Geometry check sheet. Reference: the model listing, model coordinates, mm. Round coordinates to 2 decimals unless told otherwise and drop trailing zeros. Write each loop counter-clockwise with the first axis right and the second up, starting at its lowest first coordinate (ties: lowest second). Pieces come first, ordered by that corner, then holes. Notation, with made-up numbers: (15.25, 15) -> (50.25, 15) arc R16 cw to (50.25, 45) -> close; hole circle Ø8 at (71, 17.5). An arc over 180 degrees is marked (long way). Use a Markdown table: item, result.
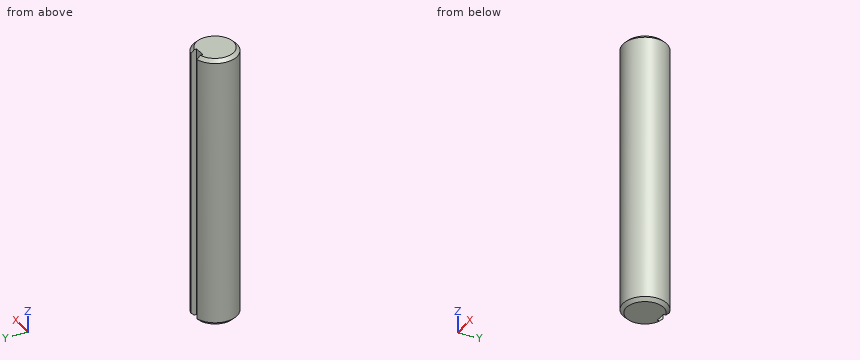
```python
from build123d import *

# Parameters (mm, degrees)
SKETCH1_R           = 4
EXTRUDE1_DEPTH      = 25
CHAMFER1_SIZE       = 0.6
SKETCH3_W           = 2
SKETCH3_H           = 1.2
EXTRUDE2_DEPTH      = 26
EXTRUDE2_DEPTH_BACK = 26


with BuildPart() as part:
    # Sketch1 → Extrude1 (new body, symmetric)
    with BuildSketch(Plane.XY):
        Circle(SKETCH1_R)
    extrude(amount=EXTRUDE1_DEPTH, both=True)

    # Chamfer1
    chamfer1_edges = [part.edges().sort_by_distance(p)[0] for p in [
        (-4, 0, -25),
        (-4, 0, 25),
    ]]
    chamfer(chamfer1_edges, length=CHAMFER1_SIZE)

    # Sketch3 → Extrude2 (cut, two sides)
    with BuildSketch(Plane.XY) as extrude2_sk:
        with Locations((0, 3.4)):
            Rectangle(SKETCH3_W, SKETCH3_H)
    extrude(amount=EXTRUDE2_DEPTH, mode=Mode.SUBTRACT)
    extrude(extrude2_sk.sketch, amount=-EXTRUDE2_DEPTH_BACK, mode=Mode.SUBTRACT)


solid = part.part
```
(1) Section check B-B on z = -8. Record the cut outline in (x, y).
A:
| item | result |
|---|---|
| outline | (-1, 2.8) -> (-1, 3.87) arc R4 ccw (long way) to (1, 3.87) -> (1, 2.8) -> close |
(2) Thickness scan on line 1 (Y direction, x = 0.25, z = 20); line 2 (X direction, y = -1, z = -6); line 3 (X direction, y = 3, z = -21.5). Record the ranges inside material, lowest first.
A:
| item | result |
|---|---|
| line 1 | y = -3.99 to 2.8 |
| line 2 | x = -3.87 to 3.87 |
| line 3 | x = -2.65 to -1, 1 to 2.65 |
(3) Gauge pin test, flat ends, axial feed: pin 1 Ø1.5 at (y, z) = (-2.5, 17) entering from -X; pin 2 Ø3 at (y, z) = (-3, -14.5) entering from +X; pin 3 Ø1.2 at (y, z) = (3.5, -2) entering from -X (3 decimals). Record the tip position at first contact, or that the pin passes through.
A:
| item | result |
|---|---|
| pin 1 | stops at x = -3.6 |
| pin 2 | stops at x = 3.71 |
| pin 3 | stops at x = -2.755 |
(4) Section check A-A on x = 0. Record the cut outline in (y, z), plus the area to 3 significant figures.
A:
| item | result |
|---|---|
| outline | (-4, -24.4) -> (-3.4, -25) -> (2.8, -25) -> (2.8, 25) -> (-3.4, 25) -> (-4, 24.4) -> close |
| area | 340 mm2 |
